Verification items for the finished model (mm, model axes). Face numbers are marked on the shaded views. Give positions to 0.01 mm unless a question says otherwise; leave off trailing zeros. Write each loop counter-clockwise with the first axis right and the second up, starting at its lowest first coordinate (ties: lowest second). Pieces come first, ordered by that corner, then holes.
from build123d import *

# Parameters (mm, degrees)
F0_W      = 12.7
F0_H      = 19.05
F1_DEPTH  = 12.7
F2_W      = 12.7
F2_H      = 19.05
F3_DEPTH  = 12.7
F4_SIZE   = 9.52499
F5_SIZE   = 6.35
F5_SIZE_2 = 6.34999
F6_R      = 6.35
F7_DEPTH  = 12.7


# Not quite as in the source:
# - a fillet or chamfer is up to 0.001 mm smaller than in the source, because OpenCascade refuses the exact size


with BuildPart() as f1:
    # F0 (on Front) → F1 (new body, symmetric)
    with BuildSketch(Plane.XZ):
        Rectangle(F0_W, F0_H)
    extrude(amount=F1_DEPTH, both=True)

    # F2 (on face) → F3 (join)
    with BuildSketch(Plane.XZ.offset(12.7)):
        Rectangle(F2_W, F2_H)
    extrude(amount=F3_DEPTH)

    # F4 (size 9.525 in the source; OpenCascade refuses exactly that, so slightly less here)
    f4_edges = [f1.edges().sort_by_distance(p)[0] for p in [
        (0, -25.4, 9.525),
        (0, -25.4, -9.525),
    ]]
    chamfer(f4_edges, length=F4_SIZE)

    # F5 (call 1 of 4: OpenCascade refuses the feature's edges together)
    f5_edges = [f1.edges().sort_by_distance(p)[0] for p in [
        (-6.35, -20.637505, 4.762505),
    ]]
    chamfer(f5_edges, length=F5_SIZE)

    # F5#2 (call 2 of 4)
    f5_2_edges = [f1.edges().sort_by_distance(p)[0] for p in [
        (-6.35, -20.637505, -4.762505),
    ]]
    chamfer(f5_2_edges, length=F5_SIZE)

    # F5#3 (call 3 of 4) (size 6.35 in the source; OpenCascade refuses exactly that, so slightly less here)
    f5_3_edges = [f1.edges().sort_by_distance(p)[0] for p in [
        (6.35, -20.637505, 4.762505),
    ]]
    chamfer(f5_3_edges, length=F5_SIZE_2)

    # F5#4 (call 4 of 4) (size 6.35 in the source; OpenCascade refuses exactly that, so slightly less here)
    f5_4_edges = [f1.edges().sort_by_distance(p)[0] for p in [
        (6.35, -20.637505, -4.762505),
    ]]
    chamfer(f5_4_edges, length=F5_SIZE_2)

    # F6 (on face) → F7 (cut)
    with BuildSketch(Plane.YZ.offset(6.35)):
        with Locations((1.27, 0)):
            Circle(F6_R)
    extrude(amount=-F7_DEPTH, mode=Mode.SUBTRACT)


solid = f1.part
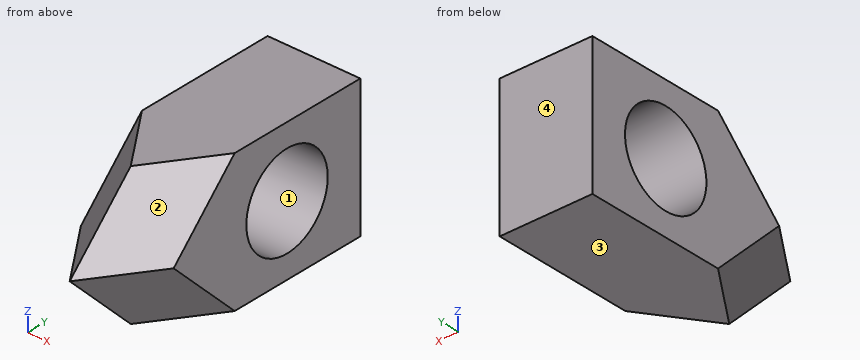
Item 1: Release check for a two-part mould opening along Y. For the marked faces 1, 2, 3 and 4 record: released by +Y, released by -Y, zero draft, split by the parting line, or undercut.
Answer key:
face 1: undercut
face 2: released by -Y
face 3: zero draft
face 4: released by +Y
Item 2: Sectioned sample at A-A on y = 1.27. Record the cut outline in (x, z) (3 decimals).
Answer key:
outline: (-6.35, -9.525) - (6.35, -9.525) - (6.35, -6.35) - (-6.35, -6.35) - close; (-6.35, 6.35) - (6.35, 6.35) - (6.35, 9.525) - (-6.35, 9.525) - close
Item 3: Scan lines: line 1 along Z through (x, y) = (0, 1.27) (3 decimals); line 2 along Y through (x, z) = (1.5, -5.25); line 3 along Y through (x, z) = (3.5, -4.5). Record each from-to range of solid material in increasing order.
Answer key:
line 1: z = -9.525 to -6.35, 6.35 to 9.525
line 2: y = -18.03 to -2.3, 4.84 to 12.7
line 3: y = -15.95 to -3.21, 5.75 to 12.7
Item 4: Depth check by flat-ended pin: pin 1 (1.5 mm diameter, centred on x = -1, y = -18.5, fed in from -Z); pin 2 (3 mm diameter, centred on x = 4.5, z = -5, fed in from -Y); pin 3 (2 mm diameter, centred on y = -19, z = -6.5, fed in from -X). Enter the tip coordinate at first touch or a pass-through.
Answer key:
pin 1: stops at z = -6.78
pin 2: stops at y = -16.63
pin 3: stops at x = -0.93
Item 5: Sectioned sample at C-C on x = 5.25. Record the cut outline in (y, z) (3 decimals), then the cut area to 3 significant figures.
Answer key:
outline: (-17.975, 0) - (-8.45, -9.525) - (12.7, -9.525) - (12.7, 9.525) - (-8.45, 9.525) - close; hole circle Ø12.7 at (1.27, 0)
area: 367 mm2
